The drawing under review shows one solid part. Ordinate dimensions are in mm from its lowest x, y, z. A direction names the side the tool comes from. Coordinates: 2 decimals unless noted, no trailing zeros. Order: outer loops, then holes, each group sorted by start corner. A loop starts at its lowest first (then second) coordinate and runs counter-clockwise, first axis right, second up. Notation, with made-up numbers: (-28.5, 26) -> (24.5, 26) arc R17 cw to (24.5, 56) -> close; hole circle Ø11 at (81.5, -30.75). An arc over 180 degrees is marked (long way). Put each result on its own line as item: value.
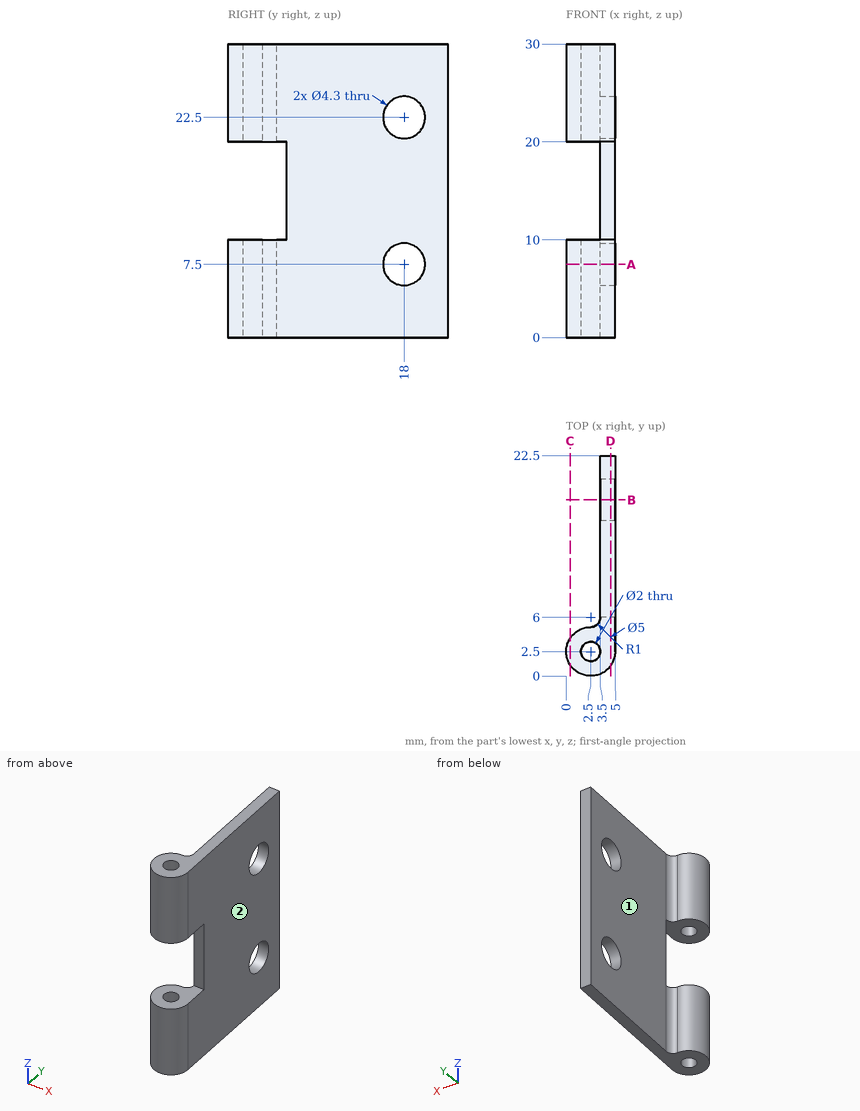
Item 1: Consider section B-B on y = 18. Write out the cut boundary in (x, z), and give its area (3 significant figures).
Answers below:
outline: (3.5, 0) -> (5, 0) -> (5, 5.35) -> (3.5, 5.35) -> close; (3.5, 9.65) -> (5, 9.65) -> (5, 20.35) -> (3.5, 20.35) -> close; (3.5, 24.65) -> (5, 24.65) -> (5, 30) -> (3.5, 30) -> close
area: 32.1 mm^2
Item 2: For pin 1 Ø8 at (y, z) = (16, 12) entering from -X; pin 2 Ø1.2 at (x, y) = (2.5, 2.5) entering from +Z; pin 3 Ø5 at (y, z) = (6, 9.5) entering from -X; pin 4 Ø0.5 at (x, z) = (4.5, 16) entering from -Y, all flat-tipped, find the tip position at first contact; note any pin that passes through.
Answers below:
pin 1: x = 3.5
pin 2: through
pin 3: x = 0.21
pin 4: y = 6
Item 3: Consider section C-C on x = 0.4. Write out the cut boundary in (y, z), and give its area (3 significant figures).
Answers below:
outline: (1.14, 0) -> (3.86, 0) -> (3.86, 10) -> (1.14, 10) -> close; (1.14, 20) -> (3.86, 20) -> (3.86, 30) -> (1.14, 30) -> close
area: 54.3 mm^2
Item 4: For line 1 (Z direction, x = 4.45, y = 18); line 2 (Z direction, x = 4.7, y = 4); line 3 (X direction, y = 8, z = 24.5), list the stretches that pass through material, from the lowest coordinate up. Write a range as from..to.
Answers below:
line 1: 0..5.35, 9.65..20.35, 24.65..30
line 2: 0..10, 20..30
line 3: 3.5..5
Item 5: For the marked faces 1 and 2, list the 3-axis set-ups (+Z, -Z, +X, -X, +Y, -Y) from which the entire face can be reached by the end or side of a thin tool; tool diameter is ignored.
Answers below:
face 1: +Z, -Z, -X, +Y
face 2: +Z, -Z, +X, +Y, -Y
Item 6: Consider section D-D on x = 4.55. Write out the cut boundary in (y, z).
Answers below:
outline: (1.07, 0) -> (22.5, 0) -> (22.5, 30) -> (1.07, 30) -> (1.07, 20) -> (6, 20) -> (6, 10) -> (1.07, 10) -> close; hole circle Ø4.3 at (18, 7.5); hole circle Ø4.3 at (18, 22.5)
Item 7: Consider section A-A on z = 7.5. Write out the cut boundary in (x, y), and give its area (3 significant figures).
Answers below:
outline: (2.5, 5) arc R2.5 ccw (long way) to (5, 2.5) -> (5, 15.85) -> (3.5, 15.85) -> (3.5, 6) arc R1 cw to start; (3.5, 20.15) -> (5, 20.15) -> (5, 22.5) -> (3.5, 22.5) -> close; hole circle Ø2 at (2.5, 2.5)
area: 37.8 mm^2
